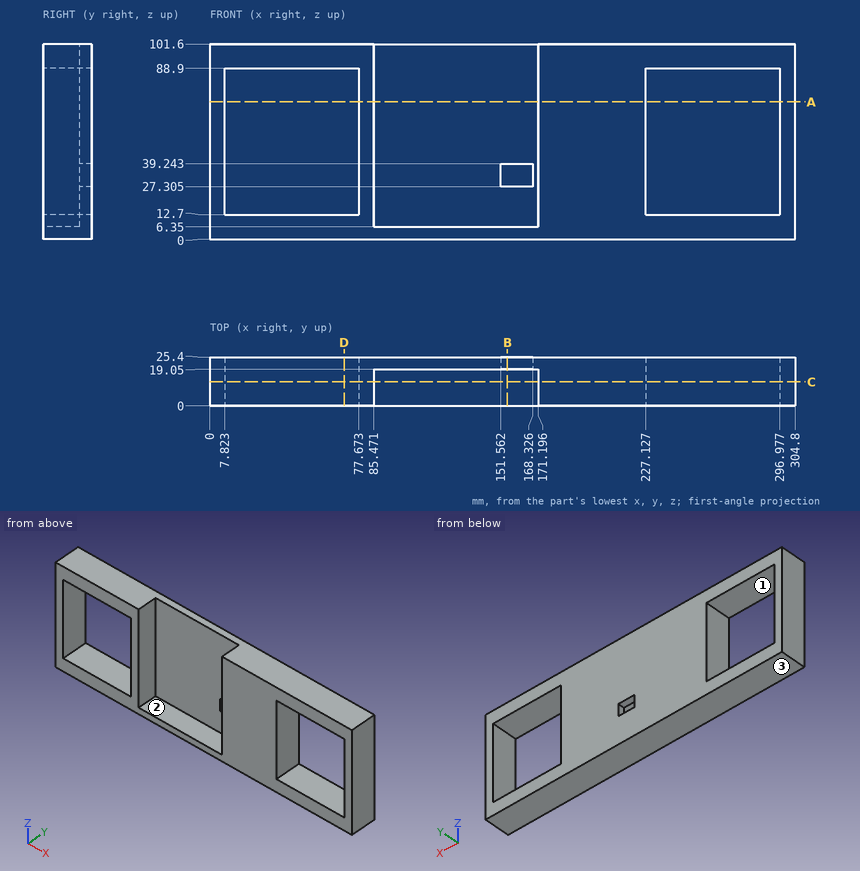
Here's the drawing with two shaded views (mm, measured from the low corner). I have some questions. A direction names the side the tool comes from. Give positions to 0.01 mm unless a question says otherwise; leave off trailing zeros. Loops run counter-clockwise (first coordinate to the right, second up) from the corner with the lowest first, then second, coordinate; pieces in that order, holes last. Notation, with made-up numbers: (21.5, 38.5) - (50.5, 38.5) arc R34 ccw to (50.5, 70.5) - close; hole circle Ø4 at (-15.75, 37). An arc over 180 degrees is marked (long way). Return JSON: item names as keys, results as strings.
1. I want a section at C-C on y = 12.5. Please give me the cut outline in (x, z).
Output values:
{"outline": "(0, 0) - (304.8, 0) - (304.8, 101.6) - (171.2, 101.6) - (171.2, 6.35) - (85.47, 6.35) - (85.47, 101.6) - (0, 101.6) - close; hole (7.82, 12.7) - (77.67, 12.7) - (77.67, 88.9) - (7.82, 88.9) - close; hole (227.13, 12.7) - (296.98, 12.7) - (296.98, 88.9) - (227.13, 88.9) - close"}
2. For the marked faces 1, 2 and 3, which set-ups out of +Z, -Z, +X, -X, +Y, -Y let a thin tool reach every point of the face, with its end or its side?
Output values:
{"face 1": "+Y, -Y", "face 2": "+Z, -Y", "face 3": "-Z, +X, -X, +Y, -Y"}
3. I'm going to push flat-ended pins straight in: pin 1 Ø4 at (x, z) = (81, 16) entering from -Y; pin 2 Ø1 at (x, y) = (113.5, 10) entering from +Z. Where does each tip first touch, or does it pass through?
Output values:
{"pin 1": "stops at y = 0", "pin 2": "stops at z = 6.35"}
4. I want a section at A-A on z = 71.5. Please give me the cut outline in (x, y).
Output values:
{"outline": "(0, 0) - (7.82, 0) - (7.82, 25.4) - (0, 25.4) - close; (77.67, 0) - (85.47, 0) - (85.47, 19.05) - (171.2, 19.05) - (171.2, 0) - (227.13, 0) - (227.13, 25.4) - (77.67, 25.4) - close; (296.98, 0) - (304.8, 0) - (304.8, 25.4) - (296.98, 25.4) - close"}
5. I want a section at B-B on x = 155. Please give me the cut outline in (y, z) (3 decimals).
Output values:
{"outline": "(0, 0) - (25.4, 0) - (25.4, 27.305) - (19.05, 27.305) - (19.05, 6.35) - (0, 6.35) - close; (19.05, 39.243) - (25.4, 39.243) - (25.4, 101.6) - (19.05, 101.6) - close"}
6. If I drill on line 1 (X direction, y = 15.5, z = 81); line 2 (X direction, y = 19.5, z = 42.5); line 3 (Z direction, x = 44, y = 11.5), over which ranges is the centre line in solid material (lowest first)?
Output values:
{"line 1": "x = 0 to 7.82, 77.67 to 85.47, 171.2 to 227.13, 296.98 to 304.8", "line 2": "x = 0 to 7.82, 77.67 to 227.13, 296.98 to 304.8", "line 3": "z = 0 to 12.7, 88.9 to 101.6"}
7. I want a section at D-D on x = 70. Please give me the cut outline in (y, z), and give its area (3 significant figures).
Output values:
{"outline": "(0, 0) - (25.4, 0) - (25.4, 12.7) - (0, 12.7) - close; (0, 88.9) - (25.4, 88.9) - (25.4, 101.6) - (0, 101.6) - close", "area": "645 mm²"}
